For this review, take the finished solid that the model builds, in its own axes (mm). Face numbers are marked on the shaded views. Give positions to 0.01 mm unless a question says otherwise; leave off trailing zeros. Write each loop counter-clockwise with the first axis right and the second up, starting at its lowest first coordinate (ties: lowest second). Pieces come first, ordered by that corner, then holes. Notation, with made-up numbers: (39.5, 83) -> (62.5, 83) arc R14 ccw to (62.5, 92) -> close; hole circle Ø5 at (48, 41.5). An arc over 180 degrees is marked (long way). Write item = value, one per line.
```python
from build123d import *

# Parameters (mm, degrees)
ESTRUSIONE_ESTRUSIONE1_DEPTH         = 42
FORO_FILETTATO_M18X1_5_1_D           = 16.5
FORO_FILETTATO_M18X1_5_1_DEPTH       = 38.542899893
FORO_FILETTATO_M18X1_5_1_CSINK_D     = 18.05
FORO_FILETTATO_M18X1_5_1_CSINK_ANGLE = 82
FORO_FILETTATO_M18X1_5_1_TIP         = 4.957100107


with BuildPart() as part:
    # Schizzo1 → Estrusione-Estrusione1 (new body)
    with BuildSketch(Plane(origin=(0, 0, 0), x_dir=(0, 0, -1), z_dir=(1, 0, 0))):
        Polygon((-30, 50), (-30, 0), (30, 0), (30, 30), (-15, 50), align=None)
    extrude(amount=ESTRUSIONE_ESTRUSIONE1_DEPTH)

    # Foro filettato M18x1.5-1
    with Locations(Plane.XY.offset(30)):
        with Locations((21, 25)):
            CounterSinkHole(FORO_FILETTATO_M18X1_5_1_D / 2, FORO_FILETTATO_M18X1_5_1_CSINK_D / 2, depth=FORO_FILETTATO_M18X1_5_1_DEPTH, counter_sink_angle=FORO_FILETTATO_M18X1_5_1_CSINK_ANGLE)
            with Locations((0, 0, -(FORO_FILETTATO_M18X1_5_1_DEPTH + FORO_FILETTATO_M18X1_5_1_TIP / 2))):  # 118° drill point
                Cone(0, FORO_FILETTATO_M18X1_5_1_D / 2, FORO_FILETTATO_M18X1_5_1_TIP, mode=Mode.SUBTRACT)


solid = part.part
```
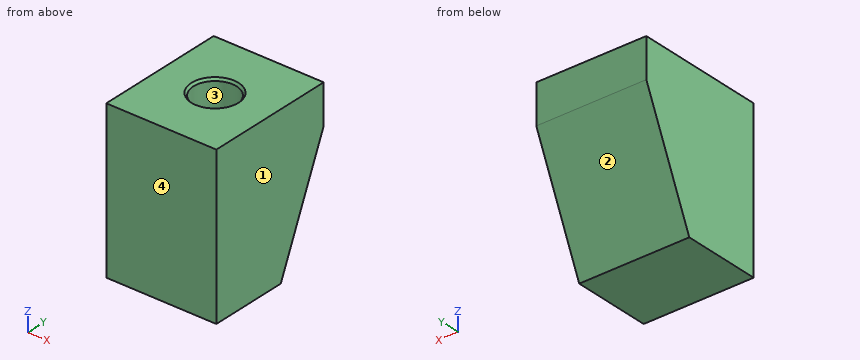
(1) The part is to be moulded in two halves that separate along Y. For the marked faces 1, 2, 3 and 4, say which applies: released by +Y, released by -Y, zero draft, split by the parting line, or undercut.
Answers below:
face_1 = zero draft
face_2 = released by +Y
face_3 = undercut
face_4 = released by -Y
(2) To check wall thickness, follow probe 1 along X at (y, z) = (25, 11); probe 2 along Y at (x, z) = (21, 9); probe 3 along Y at (x, z) = (21, 15). State the ranges of each line that lie inside material, in increasing order.
Answers below:
probe_1 = 0 to 12.75, 29.25 to 42
probe_2 = 0 to 16.75, 33.25 to 47.33
probe_3 = 0 to 16.75, 33.25 to 50
(3) Take a section at C-C (x = 34). Write out the cut boundary in (y, z), plus the area to 3 significant figures.
Answers below:
outline = (0, -30) -> (30, -30) -> (50, 15) -> (50, 30) -> (0, 30) -> close
area = 2,550 mm^2
(4) Take a section at A-A (z = -7.5). Write out the cut boundary in (x, y).
Answers below:
outline = (0, 0) -> (42, 0) -> (42, 40) -> (0, 40) -> close; hole circle Ø16.5 at (21, 25)
(5) For pin 1 (12 mm diameter, centred on x = 21, z = 15.5, fed in from -Y); pin 2 (10 mm diameter, centred on x = 21, y = 25, fed in from +Z); pin 3 (3 mm diameter, centred on x = 27, y = 43, fed in from -Z) (3 decimals); pin 4 (2 mm diameter, centred on x = 5, z = -10.5, fed in from +Y), all flat-tipped, find the tip position at first contact; note any pin that passes through.
Answers below:
pin_1 = 0
pin_2 = -10.5
pin_3 = -4.125
pin_4 = 39.11
(6) Take a section at D-D (z = 7). Write out the cut boundary in (x, y), plus the area to 3 significant figures.
Answers below:
outline = (0, 0) -> (42, 0) -> (42, 46.44) -> (0, 46.44) -> close; hole circle Ø16.5 at (21, 25)
area = 1,740 mm^2
(7) Take a section at B-B (y = 37). Write out the cut boundary in (x, z).
Answers below:
outline = (0, -14.25) -> (42, -14.25) -> (42, 30) -> (0, 30) -> close
